```python
from build123d import *

# Parameters (mm, degrees)
SKETCH1_R                = 11.013886191
BOSS_EXTRUDE1_DEPTH      = 8
BOSS_EXTRUDE2_DEPTH      = 5
BOSS_EXTRUDE2_DEPTH_BACK = 2
SKETCH2_W                = 38
SKETCH2_H                = 48
CUT_EXTRUDE1_DEPTH       = 51
CUT_EXTRUDE2_DEPTH       = 51


with BuildPart() as part:
    # Sketch1 → Boss-Extrude1 (new body)
    with BuildSketch(Plane.XY):
        with BuildLine():
            Line((0, -22.07294906), (-19, -22.07294906))
            Line((-19, -22.07294906), (-19, 0))
            ThreePointArc((-19, 0), (0, 19), (19, 0))
            Line((19, 0), (19, -22.07294906))
            Line((19, -22.07294906), (0, -22.07294906))
        make_face()
        Circle(SKETCH1_R, mode=Mode.SUBTRACT)
        with BuildLine():
            ThreePointArc((-11.340381057, -7.5), (-12.990381057, -5.85), (-14.640381057, -7.5))
            ThreePointArc((-14.640381057, -7.5), (-12.990381057, -9.15), (-11.340381057, -7.5))
        make_face(mode=Mode.SUBTRACT)
        with BuildLine():
            ThreePointArc((-5.35, -12.124355653), (-7, -10.474355653), (-8.65, -12.124355653))
            ThreePointArc((-8.65, -12.124355653), (-7, -13.774355653), (-5.35, -12.124355653))
        make_face(mode=Mode.SUBTRACT)
        with BuildLine():
            ThreePointArc((11.340381057, -7.5), (12.990381057, -9.15), (14.640381057, -7.5))
            ThreePointArc((14.640381057, -7.5), (12.990381057, -5.85), (11.340381057, -7.5))
        make_face(mode=Mode.SUBTRACT)
        with BuildLine():
            ThreePointArc((15.65, 0), (14, 1.65), (12.35, 0))
            ThreePointArc((12.35, 0), (14, -1.65), (15.65, 0))
        make_face(mode=Mode.SUBTRACT)
        with BuildLine():
            ThreePointArc((-1.65, 15), (0, 13.35), (1.65, 15))
            ThreePointArc((1.65, 15), (0, 16.65), (-1.65, 15))
        make_face(mode=Mode.SUBTRACT)
        with BuildLine():
            ThreePointArc((-5.35, 12.124355653), (-7, 13.774355653), (-8.65, 12.124355653))
            ThreePointArc((-8.65, 12.124355653), (-7, 10.474355653), (-5.35, 12.124355653))
        make_face(mode=Mode.SUBTRACT)
    extrude(amount=BOSS_EXTRUDE1_DEPTH)

    # Sketch2 → Boss-Extrude2 (add, two sides: drawn at the far end of the back side and taken through both)
    with BuildSketch(Plane.XZ.offset(22.07294906).offset(-BOSS_EXTRUDE2_DEPTH_BACK)):
        with Locations((0, -16)):
            Rectangle(SKETCH2_W, SKETCH2_H)
    extrude(amount=BOSS_EXTRUDE2_DEPTH + BOSS_EXTRUDE2_DEPTH_BACK)

    # Sketch3 → Cut-Extrude1 (cut)
    with BuildSketch(Plane(origin=(0, 0, 0), x_dir=(-1, 0, 0), z_dir=(0, 0, -1))):
        with BuildLine():
            Line((5.904398983, -20.07294906), (-5.904398983, -20.07294906))
            ThreePointArc((-5.904398983, -20.07294906), (0, -20.923317407), (5.904398983, -20.07294906))
        make_face()
    extrude(amount=CUT_EXTRUDE1_DEPTH, mode=Mode.SUBTRACT)

    # Sketch4 → Cut-Extrude2 (cut)
    with BuildSketch(Plane(origin=(0, -20.07294906, 0), x_dir=(1, 0, 0), z_dir=(0, 1, 0))):
        with BuildLine():
            Line((-13.7, 8.006381215), (-13.7, 4.606381215))
            ThreePointArc((-13.7, 4.606381215), (-12, 2.906381215), (-10.3, 4.606381215))
            Line((-10.3, 4.606381215), (-10.3, 8.006381215))
            ThreePointArc((-10.3, 8.006381215), (-12, 9.706381215), (-13.7, 8.006381215))
        make_face()
        with BuildLine():
            Line((-13.7, 33.006381215), (-13.7, 29.606381215))
            ThreePointArc((-13.7, 29.606381215), (-12, 27.906381215), (-10.3, 29.606381215))
            Line((-10.3, 29.606381215), (-10.3, 33.006381215))
            ThreePointArc((-10.3, 33.006381215), (-12, 34.706381215), (-13.7, 33.006381215))
        make_face()
        with BuildLine():
            Line((13.7, 33.006381215), (13.7, 29.606381215))
            ThreePointArc((13.7, 29.606381215), (12, 27.906381215), (10.3, 29.606381215))
            Line((10.3, 29.606381215), (10.3, 33.006381215))
            ThreePointArc((10.3, 33.006381215), (12, 34.706381215), (13.7, 33.006381215))
        make_face()
        with BuildLine():
            Line((13.7, 8.006381215), (13.7, 4.606381215))
            ThreePointArc((13.7, 4.606381215), (12, 2.906381215), (10.3, 4.606381215))
            Line((10.3, 4.606381215), (10.3, 8.006381215))
            ThreePointArc((10.3, 8.006381215), (12, 9.706381215), (13.7, 8.006381215))
        make_face()
    extrude(amount=-CUT_EXTRUDE2_DEPTH, mode=Mode.SUBTRACT)


solid = part.part
```
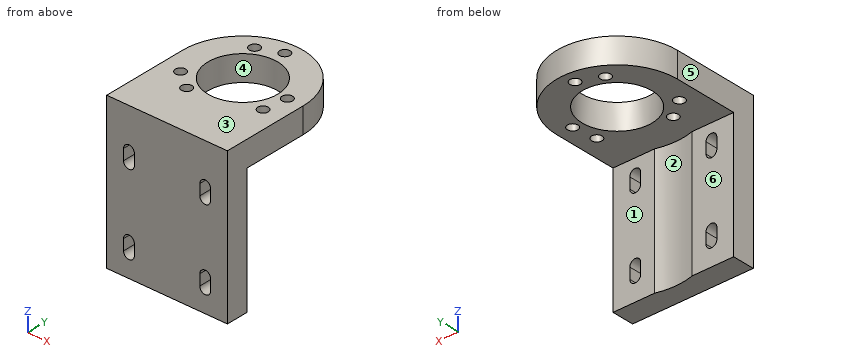
Build history of the part. All positions in model axes, mm. Face numbers are marked on the shaded views. A direction names the side the tool comes from. Coordinates: 2 decimals unless noted, no trailing zeros. Order: outer loops, then holes, each group sorted by start corner. A loop starts at its lowest first (then second) coordinate and runs counter-clockwise, first axis right, second up. Notation, with made-up numbers: M -1.5,27 L 42.5,27 A20 ccw 42.5,49 Z; hole C 85,79 d9. An arc over 180 degrees is marked long. One line per question, with ' | ' between items. Start each with the question number.
1. Cut at D-D (z = -23.5). Write the cut outline in (x, y).
2. Cut at C-C (y = -2.5). Write the cut outline in (x, z), plus the area to 3 significant figures.
3. Cut at B-B (z = -34). Write the cut outline in (x, y), plus the area to 3 significant figures.
4. Wall check: line 1 along Y through (x, z) = (0, 5); line 2 along Y through (x, z) = (-7, 5.5); line 3 along Z through (x, y) = (10, -14). Give the ranges that are in metal, low to high. Write a range as [from, to].
5. Mould opens along X. For the marked faces 4, 5 and 6 say: +X half, -X half, draft (parallel to the pull), parting line (faces both ways), or undercut.
6. Flat gauge pins, fed straight in: P1, Ø6, axis at x = 10.5, y = 7.5, coming from the -Z side; P2, Ø10.5, axis at x = -10, z = -18.5, coming from the +Y side; P3, Ø17.5, axis at x = 0, y = 0, coming from the -Z side. Where does each tip first touch, or does it go through?
7. Tool access for the marked faces 1, 2 and 3: list every direction of +Z, -Z, +X, -X, +Y, -Y with a clear straight run to the whole face (end or side of a thin tool).
8. Cut at A-A (x = -7). Write the cut outline in (y, z).
The answers:
1) outline: M -19,-27.07 L 19,-27.07 L 19,-20.07 L 5.9,-20.07 A20.92 cw -5.9,-20.07 L -19,-20.07 Z
2) outline: M -19,0 L -10.73,0 L -10.73,8 L -19,8 Z; M 10.73,0 L 19,0 L 19,8 L 10.73,8 Z | area: 132 mm2
3) outline: M -19,-27.07 L -13.38,-27.07 L -13.38,-20.07 L -19,-20.07 Z; M -10.62,-27.07 L 10.62,-27.07 L 10.62,-20.07 L 5.9,-20.07 A20.92 cw -5.9,-20.07 L -10.62,-20.07 Z; M 13.38,-27.07 L 19,-27.07 L 19,-20.07 L 13.38,-20.07 Z | area: 221 mm2
4) line 1: y = [-27.07, -11.01], [11.01, 13.35], [16.65, 19] | line 2: y = [-27.07, -13.77], [-10.47, -8.5], [8.5, 10.47], [13.77, 17.66] | line 3: z = [0, 8]
5) face 4: undercut | face 5: -X half | face 6: draft
6) P1: stops at z = 0 | P2: stops at y = -20.07 | P3: passes through
7) face 1: -Z, +X, -X, +Y | face 2: -Z, +Y | face 3: +Z, +X, -X, +Y, -Y
8) outline: M -27.07,-40 L -20.07,-40 L -20.07,0 L -13.77,0 L -13.77,8 L -27.07,8 Z; M -10.47,0 L -8.5,0 L -8.5,8 L -10.47,8 Z; M 8.5,0 L 10.47,0 L 10.47,8 L 8.5,8 Z; M 13.77,0 L 17.66,0 L 17.66,8 L 13.77,8 Z
